Check sheet for the modelled part. Datum: model origin and axes. Units: mm. A direction names the side the tool comes from. Give positions to 0.01 mm unless a question says otherwise; leave off trailing zeros. Loops run counter-clockwise (first coordinate to the right, second up) from the corner with the lowest first, then second, coordinate; pieces in that order, holes last. Notation, with made-up numbers: (38.5, 22.25) - (78.5, 22.25) arc R16 cw to (78.5, 37.25) - close; hole circle Ø2 at (-31.75, -28). An arc over 180 degrees is marked (long way). Use CSV: the item, a comma, the result in double quotes.
from build123d import *

# Parameters (mm, degrees)
SKETCH1_W               = 235
SKETCH1_H               = 40
BOSS_EXTRUDE1_DEPTH     = 4
SKETCH2_W               = 3.7
SKETCH2_H               = 20
CUT_EXTRUDE1_DEPTH      = 4
SKETCH3_R               = 10
CUT_EXTRUDE2_DEPTH      = 4
LPATTERN1_COUNT         = 8
LPATTERN1_PITCH         = 25
SKETCH4_R               = 4
CUT_EXTRUDE3_DEPTH      = 4
SKETCH5_R               = 4
BOSS_EXTRUDE2_DEPTH     = 4
MIRROR1_COPY_1_SKETCH_R = 10
MIRROR1_COPY_1_DEPTH    = 4
MIRROR1_COPY_2_SKETCH_R = 10
MIRROR1_COPY_2_DEPTH    = 4
MIRROR1_COPY_3_SKETCH_R = 10
MIRROR1_COPY_3_DEPTH    = 4
MIRROR1_COPY_4_SKETCH_R = 10
MIRROR1_COPY_4_DEPTH    = 4
MIRROR1_COPY_5_SKETCH_R = 10
MIRROR1_COPY_5_DEPTH    = 4
MIRROR1_COPY_6_SKETCH_R = 10
MIRROR1_COPY_6_DEPTH    = 4
MIRROR1_COPY_7_SKETCH_R = 10
MIRROR1_COPY_7_DEPTH    = 4


with BuildPart() as part:
    # Sketch1 → Boss-Extrude1 (new body)
    with BuildSketch(Plane(origin=(0, 0, 0), x_dir=(1, 0, 0), z_dir=(0, 1, 0))):
        with Locations((117.5, 20)):
            Rectangle(SKETCH1_W, SKETCH1_H)
    extrude(amount=BOSS_EXTRUDE1_DEPTH)

    # Sketch2 → Cut-Extrude1 (cut)
    with BuildSketch(Plane(origin=(0, 4, 0), x_dir=(1, 0, 0), z_dir=(0, 1, 0))):
        with Locations((5.85, 30)):
            Rectangle(SKETCH2_W, SKETCH2_H)
        with Locations((229.15, 30)):
            Rectangle(SKETCH2_W, SKETCH2_H)
    extrude(amount=-CUT_EXTRUDE1_DEPTH, mode=Mode.SUBTRACT)

    # Sketch3 → Cut-Extrude2 (cut)
    with BuildSketch(Plane(origin=(0, 4, 0), x_dir=(1, 0, 0), z_dir=(0, 1, 0))):
        with Locations((30, 40)):
            Circle(SKETCH3_R)
    cut_extrude2 = extrude(amount=-CUT_EXTRUDE2_DEPTH, mode=Mode.SUBTRACT)

    # LPattern1: Cut-Extrude2 ×8
    with Locations(*[(i * LPATTERN1_PITCH, 0, 0) for i in range(1, LPATTERN1_COUNT)]):
        add(cut_extrude2, mode=Mode.SUBTRACT)

    # Sketch4 → Cut-Extrude3 (cut)
    with BuildSketch(Plane(origin=(0, 4, 0), x_dir=(1, 0, 0), z_dir=(0, 1, 0))):
        with Locations((221.15, 40)):
            Circle(SKETCH4_R)
        with Locations((13.85, 40)):
            Circle(SKETCH4_R)
    extrude(amount=-CUT_EXTRUDE3_DEPTH, mode=Mode.SUBTRACT)

    # Sketch5 → Boss-Extrude2 (add)
    with BuildSketch(Plane(origin=(0, 4, 0), x_dir=(1, 0, 0), z_dir=(0, 1, 0))):
        with Locations((221.15, 0)):
            Circle(SKETCH5_R)
        with Locations((13.85, 0)):
            Circle(SKETCH5_R)
    extrude(amount=-BOSS_EXTRUDE2_DEPTH)

    # Mirror1: Cut-Extrude2 across plane
    add(cut_extrude2.mirror(Plane(origin=(0, 0, -20), x_dir=(1, 0, 0), z_dir=(0, 0, -1))), mode=Mode.SUBTRACT)

    # Mirror1 copy 1 sketch → Mirror1 copy 1 (cut)
    with BuildSketch(Plane(origin=(25, 4, -40), x_dir=(1, 0, 0), z_dir=(0, 1, 0))):
        with Locations((30, -40)):
            Circle(MIRROR1_COPY_1_SKETCH_R)
    extrude(amount=-MIRROR1_COPY_1_DEPTH, mode=Mode.SUBTRACT)

    # Mirror1 copy 2 sketch → Mirror1 copy 2 (cut)
    with BuildSketch(Plane(origin=(50, 4, -40), x_dir=(1, 0, 0), z_dir=(0, 1, 0))):
        with Locations((30, -40)):
            Circle(MIRROR1_COPY_2_SKETCH_R)
    extrude(amount=-MIRROR1_COPY_2_DEPTH, mode=Mode.SUBTRACT)

    # Mirror1 copy 3 sketch → Mirror1 copy 3 (cut)
    with BuildSketch(Plane(origin=(75, 4, -40), x_dir=(1, 0, 0), z_dir=(0, 1, 0))):
        with Locations((30, -40)):
            Circle(MIRROR1_COPY_3_SKETCH_R)
    extrude(amount=-MIRROR1_COPY_3_DEPTH, mode=Mode.SUBTRACT)

    # Mirror1 copy 4 sketch → Mirror1 copy 4 (cut)
    with BuildSketch(Plane(origin=(100, 4, -40), x_dir=(1, 0, 0), z_dir=(0, 1, 0))):
        with Locations((30, -40)):
            Circle(MIRROR1_COPY_4_SKETCH_R)
    extrude(amount=-MIRROR1_COPY_4_DEPTH, mode=Mode.SUBTRACT)

    # Mirror1 copy 5 sketch → Mirror1 copy 5 (cut)
    with BuildSketch(Plane(origin=(125, 4, -40), x_dir=(1, 0, 0), z_dir=(0, 1, 0))):
        with Locations((30, -40)):
            Circle(MIRROR1_COPY_5_SKETCH_R)
    extrude(amount=-MIRROR1_COPY_5_DEPTH, mode=Mode.SUBTRACT)

    # Mirror1 copy 6 sketch → Mirror1 copy 6 (cut)
    with BuildSketch(Plane(origin=(150, 4, -40), x_dir=(1, 0, 0), z_dir=(0, 1, 0))):
        with Locations((30, -40)):
            Circle(MIRROR1_COPY_6_SKETCH_R)
    extrude(amount=-MIRROR1_COPY_6_DEPTH, mode=Mode.SUBTRACT)

    # Mirror1 copy 7 sketch → Mirror1 copy 7 (cut)
    with BuildSketch(Plane(origin=(175, 4, -40), x_dir=(1, 0, 0), z_dir=(0, 1, 0))):
        with Locations((30, -40)):
            Circle(MIRROR1_COPY_7_SKETCH_R)
    extrude(amount=-MIRROR1_COPY_7_DEPTH, mode=Mode.SUBTRACT)


solid = part.part
1. Sectioned sample at C-C, the plane x = 200. Record the boundary of the cut face in (y, z), and give its area (3 significant figures).
Completed:
outline,"(0, -31.34) - (4, -31.34) - (4, -8.66) - (0, -8.66) - close"
area,"90.7 mm²"
2. Go/stop test with flat-tipped pins: pin 1 Ø2 at (x, y) = (231.5, 2) entering from +Z; pin 2 Ø1.1 at (x, y) = (228.5, 2) entering from -Z. Record where each tip stops, or that it passes through.
Completed:
pin 1,"stops at z = 0"
pin 2,"stops at z = -20"
3. Set-up check for faces 1 (the face through (230, 2, 0)), 2 (the face through (227.3, 2, -30)), 3 (the face through (42, 2, 0)): record each of +Z, -Z, +X, -X, +Y, -Y from which the full face is reachable in a straight line by a thin tool's end or side.
Completed:
face 1,"+Z, +X, +Y, -Y"
face 2,"-Z, +Y, -Y"
face 3,"+Z, +Y, -Y"
4. Sectioned sample at A-A, the plane z = -32. State how many separate pieces and enclosed holes the cut face has, and give its area (3 significant figures).
Completed:
separate pieces,"11"
enclosed holes,"0"
area,"526 mm²"
5. Scan lines: line 1 along X through (y, z) = (2.4, -27); line 2 along Z through (x, y) = (191.5, 1.15); line 3 along Z through (x, y) = (106.5, 1.8). Record each from-to range of solid material in increasing order.
Completed:
line 1,"x = 0 to 4, 7.7 to 227.3, 231 to 235"
line 2,"z = -40 to 0"
line 3,"z = -30.11 to -9.89"
6. Sectioned sample at B-B, the plane x = 130. Record the boundary of the cut face in (y, z).
Completed:
outline,"(0, -30) - (4, -30) - (4, -10) - (0, -10) - close"
